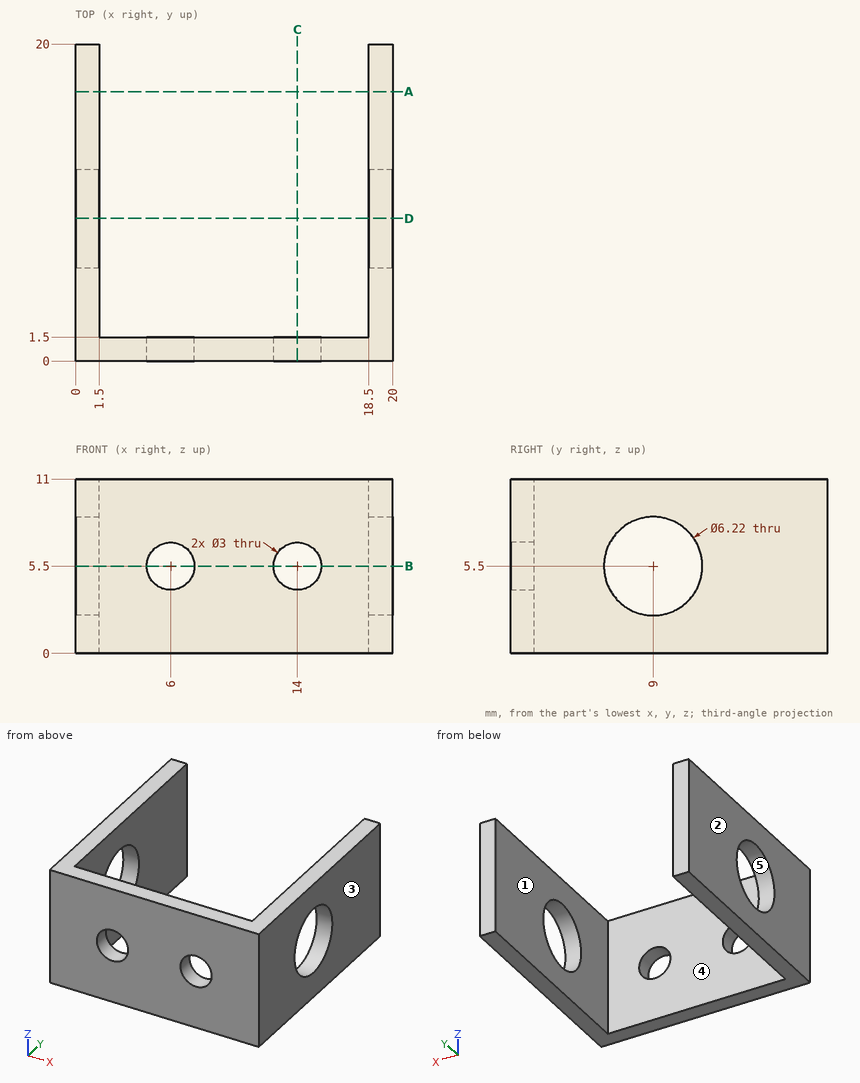
Design review of the part shown in the three views and the two pictorial views. Dimensions are in mm from the part's minimum x, y and z. A direction names the side the tool comes from. Give positions to 0.01 mm unless a question says otherwise; leave off trailing zeros. Write each loop counter-clockwise with the first axis right and the second up, starting at its lowest first coordinate (ties: lowest second). Pieces come first, ordered by that corner, then holes.
Item 1: Wall thickness on probe 1 along X at (y, z) = (19, 7.25); probe 2 along X at (y, z) = (1, 5.75); probe 3 along Y at (x, z) = (3, 2.75): over which ranges is each line inside the solid? List them lowest first.
Item 2: The part is to be moulded in two halves that separate along X. For the marked faces 3, 4 and 5, say which applies: +X half, -X half, draft (parallel to the pull), parting line (faces both ways), or undercut.
Item 3: Take a section at D-D (y = 9). Give the boundary of the cut face in (x, z).
Item 4: Take a section at C-C (x = 14). Give the boundary of the cut face in (y, z), and give its area (3 significant figures).
Item 5: Take a section at A-A (y = 17). Give the boundary of the cut face in (x, z), and give its area (3 significant figures).
Item 6: Machinability: for the marked faces 1 and 2, which of the approach directions +Z, -Z, +X, -X, +Y, -Y give a long, thin tool a straight path to every point of the face, cutting with its end or side? Answer none if there is none.
Item 7: Take a section at B-B (z = 5.5). Give the boundary of the cut face in (x, y), and give its area (3 significant figures).
Item 8: Insertion check: P1, Ø3.5, axis at x = 8, z = 5, coming from the +Y side. The pin has a flat end and moves straight along its axis. Give the tip position at first contact, or say it passes through.
Established:
1. probe 1: x = 0 to 1.5, 18.5 to 20
1. probe 2: x = 0 to 4.52, 7.48 to 12.52, 15.48 to 20
1. probe 3: y = 0 to 1.5
2. face 3: +X half
2. face 4: undercut
2. face 5: draft
3. outline: (0, 0) - (1.5, 0) - (1.5, 2.39) - (0, 2.39) - close; (0, 8.61) - (1.5, 8.61) - (1.5, 11) - (0, 11) - close; (18.5, 0) - (20, 0) - (20, 2.39) - (18.5, 2.39) - close; (18.5, 8.61) - (20, 8.61) - (20, 11) - (18.5, 11) - close
4. outline: (0, 0) - (1.5, 0) - (1.5, 4) - (0, 4) - close; (0, 7) - (1.5, 7) - (1.5, 11) - (0, 11) - close
4. area: 12.0 mm2
5. outline: (0, 0) - (1.5, 0) - (1.5, 11) - (0, 11) - close; (18.5, 0) - (20, 0) - (20, 11) - (18.5, 11) - close
5. area: 33.0 mm2
6. face 1: +Z, -Z, +Y
6. face 2: +Z, -Z, -X, +Y, -Y
7. outline: (0, 0) - (4.5, 0) - (4.5, 1.5) - (1.5, 1.5) - (1.5, 5.89) - (0, 5.89) - close; (0, 12.11) - (1.5, 12.11) - (1.5, 20) - (0, 20) - close; (7.5, 0) - (12.5, 0) - (12.5, 1.5) - (7.5, 1.5) - close; (15.5, 0) - (20, 0) - (20, 5.89) - (18.5, 5.89) - (18.5, 1.5) - (15.5, 1.5) - close; (18.5, 12.11) - (20, 12.11) - (20, 20) - (18.5, 20) - close
7. area: 57.8 mm2
8. P1: stops at y = 1.5
